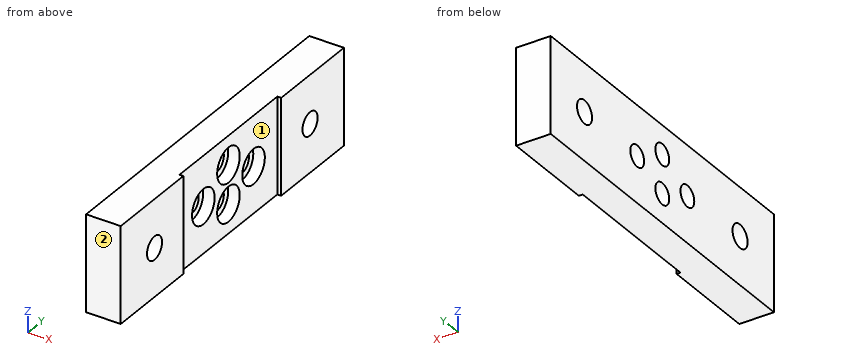
Autodesk Inventor part; units mm, degrees
ref_plane "YZ Plane" through (0, 0, 0) normal (1, 0, 0) x (0, 1, 0)
ref_plane "XZ Plane" through (0, 0, 0) normal (0, 1, 0) x (-1, 0, 0)
ref_plane "XY Plane" through (0, 0, 0) normal (0, 0, 1) x (1, 0, 0)
sketch "Sketch1" plane through (0, 0, 0) normal (0, 1, 0) x (-1, 0, 0)
  line L0 (0, 0) -> (8, 0)
  line L1 (8, 0) -> (8, -25)
  line L2 (8, -25) -> (0, -25)
  line L3 (0, -25) -> (0, 0)
  dimension "d0" = 8
  dimension "d1" = 25
extrude "Extrusion1" add sketch "Sketch1" along normal blind 89
sketch "Sketch2" plane through (0, 0, 0) normal (1, 0, 0) x (0, 0, -1)
  line L0 (0, 89) -> (25, 89)
  line L1 (0, 89) -> (25, 89)
  line L2 (25, 89) -> (25, 64)
  line L3 (25, 64) -> (0, 64)
  line L4 (0, 64) -> (0, 89)
  line L5 (25, 0) -> (25, 89)
  line L6 (25, 0) -> (0, 0)
  line L7 (0, 0) -> (0, 25)
  line L8 (0, 25) -> (25, 25)
  line L9 (25, 25) -> (25, 0)
  dimension "d4" = 25
  dimension "d5" = 25
  dimension "d6" = 25
  dimension "d7" = 25
extrude "Extrusion2" add sketch "Sketch2" along normal blind 1
sketch "Sketch3" plane through (1, 0, 0) normal (1, 0, 0) x (0, 0, -1)
  line L0 (0, 0) -> (25, 0)
  line L1 (0, 0) -> (12.5, 0)
  line L2 (12.5, 0) -> (12.5, 13.5)
  circle A0 centre (12.5, 13.5) radius 3
  circle A1 centre (12.5, 75.5) radius 3
  line L3 (25, 89) -> (0, 89)
  line L4 (0, 89) -> (0, 64)
  dimension "d10" = 13.5
  dimension "d11" = 6
  dimension "d12" = 6
  dimension "d13" = 13.5
  dimension "d14" = 12.5
sketch "Sketch4" plane through (0, 25, -25) normal (1, 0, 0) x (0, 0, -1)
  circle A0 centre (-17.5, 19.5) radius 2.75
  line L0 (-25, -25) -> (0, -25)
  line L1 (-25, 0) -> (-25, 39)
  circle A1 centre (-7.5, 19.5) radius 2.75
  line L2 (0, 0) -> (0, 39)
  circle A2 centre (-12, 9.5) radius 2.75
  circle A3 centre (-12, 29.5) radius 2.75
  dimension "d15" = 5.5
  dimension "d16" = 44.5
  dimension "d17" = 7.5
  dimension "d18" = 5.5
  dimension "d19" = 7.5
  dimension "d20" = 44.5
  dimension "d21" = 5.5
  dimension "d22" = 5.5
  dimension "d23" = 10
  dimension "d24" = 4.5
  dimension "d25" = 10
  dimension "d26" = 4.5
extrude "Extrusion3" cut sketch "Sketch3" against normal up to next
extrude "Extrusion4" cut sketch "Sketch4" against normal up to next
sketch "Sketch6" plane through (0, 25, -25) normal (1, 0, 0) x (0, 0, -1)
  circle A0 centre (-12, 29.5) radius 2.75
  circle A1 centre (-12, 29.5) radius 2.5
  circle A2 centre (-7.5, 19.5) radius 2.75
  circle A3 centre (-7.5, 19.5) radius 2.5
  circle A4 centre (-12, 9.5) radius 2.75
  circle A5 centre (-12, 9.5) radius 2.5
  circle A6 centre (-17.5, 19.5) radius 2.75
  circle A7 centre (-17.5, 19.5) radius 2.5
  circle A8 centre (-17.5, 19.5) radius 4.5
  circle A9 centre (-12, 29.5) radius 4.5
  circle A10 centre (-12, 9.5) radius 4.5
  circle A11 centre (-7.5, 19.5) radius 4.5
  point P0 (-25, -25)
  dimension "d37" = 9
  dimension "d38" = 9
  dimension "d39" = 9
  dimension "d40" = 5.5
  dimension "d41" = 5.5
  dimension "d43" = 9
extrude "Extrusion6" cut sketch "Sketch6" against normal blind 3 contours A8 | A9 | A10 | A11
properties part number "Back_Bracket_40mm" material "ABS Plastic"
Part model, mm, in its own coordinate system. Face numbers are marked on the shaded views. A direction names the side the tool comes from. Coordinates: 2 decimals unless noted, no trailing zeros. Loops run counter-clockwise (first coordinate to the right, second up) from the corner with the lowest first, then second, coordinate; pieces in that order, holes last. Notation, with made-up numbers: (-7.5, 13) -> (50.5, 13) arc R29 cw to (50.5, 42) -> close; hole circle Ø5 at (49, 32). An arc over 180 degrees is marked (long way). Use a Markdown table: item, result. Add a question column.
Item 1: Band-saw the part on C-C on z = -7.5. Write the cut outline in (x, y).
Item 2: Flat gauge pins, fed straight in: P1, Ø10.5, axis at y = 44.5, z = -7.5, coming from the +X side; P2, Ø5, axis at y = 44.5, z = -7.5, coming from the -X side; P3, Ø4.5, axis at y = 55.5, z = -11.5, coming from the +X side. Where does each tip first touch, or does it go through?
Item 3: Band-saw the part on A-A on y = 34.5. Write the cut outline in (x, z).
Item 4: Band-saw the part on B-B on x = -6.5. Write the cut outline in (y, z), plus the area to 3 significant figures.
Item 5: Band-saw the part on D-D on y = 75.5. Write the cut outline in (x, z), plus the area to 3 significant figures.
Item 6: Probe probe 1 along Z at (x, y) = (-2.75, 48); probe 2 along Z at (x, y) = (-0.5, 47.5); probe 3 along Y at (x, z) = (-0.5, -5.5). List the from-to ranges inside material, lowest first.
Item 7: Which spindle directions (+Z, -Z, +X, -X, +Y, -Y) get a long thin tool onto all of the face, cutting with end or side? Do the marked faces 1 and 2. Say none if no direction does.
Geometry says:
| question | item | result |
|---|---|---|
| 1 | outline | (-8, 0) -> (1, 0) -> (1, 25) -> (0, 25) -> (0, 40) -> (-3, 40) -> (-3, 41.75) -> (-8, 41.75) -> close; (-8, 47.25) -> (-3, 47.25) -> (-3, 49) -> (0, 49) -> (0, 64) -> (1, 64) -> (1, 89) -> (-8, 89) -> close |
| 2 | P1 | x = 0 |
| 2 | P2 | through |
| 2 | P3 | x = -3 |
| 3 | outline | (-8, -25) -> (0, -25) -> (0, -17.5) -> (-3, -17.5) -> (-3, -15.75) -> (-8, -15.75) -> close; (-8, -10.25) -> (-3, -10.25) -> (-3, -8.5) -> (0, -8.5) -> (0, 0) -> (-8, 0) -> close |
| 4 | outline | (0, -25) -> (89, -25) -> (89, 0) -> (0, 0) -> close; hole circle Ø6 at (13.5, -12.5); hole circle Ø5.5 at (34.5, -13); hole circle Ø5.5 at (44.5, -17.5); hole circle Ø5.5 at (44.5, -7.5); hole circle Ø5.5 at (54.5, -13); hole circle Ø6 at (75.5, -12.5) |
| 4 | area | 2,070 mm² |
| 5 | outline | (-8, -25) -> (1, -25) -> (1, -15.5) -> (-8, -15.5) -> close; (-8, -9.5) -> (1, -9.5) -> (1, 0) -> (-8, 0) -> close |
| 5 | area | 171 mm² |
| 6 | probe 1 | -25 to -20.33, -14.67 to -10.33, -4.67 to 0 |
| 6 | probe 2 | -25 to -20.85, -14.15 to -10.85, -4.15 to 0 |
| 6 | probe 3 | 0 to 40.47, 48.53 to 89 |
| 7 | face 1 | +Z, -Z, +X |
| 7 | face 2 | +Z, -Z, +X, -X, -Y |
